from build123d import *

# Parameters (mm, degrees)
SKETCH1_R           = 4
BOSS_EXTRUDE1_DEPTH = 10


with BuildPart() as part:
    # Sketch1 → Boss-Extrude1 (new body)
    with BuildSketch(Plane.XY):
        with BuildLine():
            Line((-62.5, 12.5), (57.5, 12.5))
            ThreePointArc((57.5, 12.5), (61.035533906, 11.035533906), (62.5, 7.5))
            Line((62.5, 7.5), (62.5, -7.5))
            ThreePointArc((62.5, -7.5), (61.035533906, -11.035533906), (57.5, -12.5))
            Line((57.5, -12.5), (-62.5, -12.5))
            Line((-62.5, -12.5), (-62.5, -8.35))
            ThreePointArc((-62.5, -8.35), (-54.15, 0), (-62.5, 8.35))
            Line((-62.5, 8.35), (-62.5, 12.5))
        make_face()
        with Locations((53.5, 0)):
            Circle(SKETCH1_R, mode=Mode.SUBTRACT)
    extrude(amount=BOSS_EXTRUDE1_DEPTH)


solid = part.part
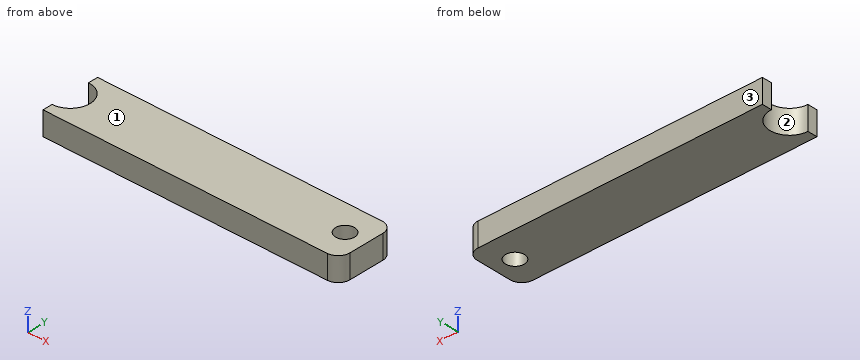
CAD build for the part. Positions are in the model's coordinates, mm. Face numbers are marked on the shaded views. Give positions to 0.01 mm unless a question says otherwise; leave off trailing zeros. Write each loop counter-clockwise with the first axis right and the second up, starting at its lowest first coordinate (ties: lowest second). Pieces come first, ordered by that corner, then holes. Notation, with made-up numbers: (41, 69.5) - (52, 69.5) arc R14 cw to (52, 94.5) - close; hole circle Ø9 at (-30, -39.75). An arc over 180 degrees is marked (long way). Put each result on its own line as item: value.
(1) Saw through at B-B (x = 53.5). List the corners of the cut face in (y, z).
Working result:
outline: (-12.5, 0) - (-4, 0) - (-4, 10) - (-12.5, 10) - close; (4, 0) - (12.5, 0) - (12.5, 10) - (4, 10) - close
(2) Pull direction Y, two halves, no side cores. Call the marked faces 1, 2 and 3: released by +Y, released by -Y, zero draft, split by the parting line, or undercut.
Working result:
face 1: zero draft
face 2: undercut
face 3: released by +Y
(3) Wall check: L1, parallel to Y at x = 53.5, z = 6.25; L2, parallel to X at y = -2, z = 4.25; L3, parallel to X at y = 1.5, z = 7.75. Give the ranges that are in metal, low to high.
Working result:
L1: -12.5 to -4, 4 to 12.5
L2: -54.39 to 50.04, 56.96 to 62.5
L3: -54.29 to 49.79, 57.21 to 62.5
(4) Saw through at D-D (y = 5.75). List the corners of the cut face in (x, z), then the cut area to 3 significant figures.
Working result:
outline: (-56.45, 0) - (62.5, 0) - (62.5, 10) - (-56.45, 10) - close
area: 1,190 mm^2
(5) Saw through at C-C (z = 5.25). List the corners of the cut face in (x, y), then the cut area to 3 significant figures.
Working result:
outline: (-62.5, -12.5) - (57.5, -12.5) arc R5 ccw to (62.5, -7.5) - (62.5, 7.5) arc R5 ccw to (57.5, 12.5) - (-62.5, 12.5) - (-62.5, 8.35) arc R8.35 cw to (-62.5, -8.35) - close; hole circle Ø8 at (53.5, 0)
area: 2,950 mm^2
(6) Saw through at A-A (y = 0). List the corners of the cut face in (x, z), then the cut area to 3 significant figures.
Working result:
outline: (-54.15, 0) - (49.5, 0) - (49.5, 10) - (-54.15, 10) - close; (57.5, 0) - (62.5, 0) - (62.5, 10) - (57.5, 10) - close
area: 1,090 mm^2
